For this review, take the finished solid that the model builds, in its own axes (mm). A direction names the side the tool comes from. Round coordinates to 2 decimals unless told otherwise and drop trailing zeros. Write each loop counter-clockwise with the first axis right and the second up, starting at its lowest first coordinate (ties: lowest second). Pieces come first, ordered by that corner, then holes. Notation, with made-up numbers: M 75,13.5 L 120,13.5 A18 ccw 120,20.5 Z; hole C 85,22.5 d2. An arc over 180 degrees is marked long. Use one line per item in the form item = value. Start each with the question number.
Item 1: Add section B-B (x = -9.5). State the section outline as (y, z) points.
Item 2: For P1, Ø0.8, axis at x = -20.5, z = 14.5, coming from the +Y side; P2, Ø1.5, axis at y = 2.5, z = -13.5, coming from the -X side; P3, Ø10, axis at x = -28, z = 1.5, coming from the +Y side, all flat-tipped, find the tip position at first contact; note any pin that passes through.
Item 3: For line 1 (X direction, y = 3.05, z = -2); line 2 (Z direction, x = -24.5, y = 2.1); line 3 (X direction, y = 1, z = 6), list the stretches that pass through material, from the lowest coordinate up. Write a range as [from, to].
Item 4: For faces 1 (the conical face through (-46.59, 0.54, -13.7)), 2 (the cylindrical face through (-45.4, 2.24, 15.12)), 3 (the flat face through (-20, 3, -15)), list the 3-axis set-ups (+Z, -Z, +X, -X, +Y, -Y) from which the entire face can be reached by the end or side of a thin tool; tool diameter is ignored.
Item 5: Add section A-A (z = 1). State the section outline as (x, y) points.
Item 6: Draft analysis for pull direction X (two halves, no side actions). For faces 4 (the flat face through (-49.01, 0.96, -0.14)), 5 (the flat face through (-2, 2, -0.15)), 6 (the flat face through (-21, 3, -17)), state which applies: released by +X, released by -X, zero draft, split by the parting line, or undercut.
from build123d import *

# Parameters (mm, degrees)
BOSS_EXTRUDE1_DEPTH     = 42
SKETCH3_W               = 4.5
SKETCH3_H               = 0.7
BOSS_EXTRUDE2_DEPTH     = 1.899999
SKETCH6_W               = 2.500000024
SKETCH6_H               = 0.3
REVOLVE1_ANGLE          = 90
SKETCH7_W               = 2.7
SKETCH7_H               = 5
BOSS_EXTRUDE3_DEPTH     = 2.50000008
SKETCH9_W               = 3.499999976
SKETCH9_H               = 5
CUT_EXTRUDE1_DEPTH      = 1.50000008
SKETCH10_W              = 0.3
SKETCH10_H              = 5
REVOLVE2_ANGLE          = 90
BOSS_EXTRUDE5_START     = -5
BOSS_EXTRUDE5_DEPTH     = 5
REVOLVE4_ANGLE          = 90
REVOLVE6_ANGLE          = 90
BOSS_EXTRUDE7_DEPTH     = 18
BOSS_EXTRUDE8_DEPTH     = 2.9
CUT_EXTRUDE2_DEPTH      = 2.9
BOSS_EXTRUDE9_START     = -1.899999
BOSS_EXTRUDE9_DEPTH     = 1.899999
SKETCH29_W              = 3
SKETCH29_H              = 0.9
BOSS_EXTRUDE10_DEPTH    = 1.3
CUT_EXTRUDE3_START      = -3.1
CUT_EXTRUDE3_DEPTH      = 3.1
CUT_EXTRUDE4_START      = -44.9
CUT_EXTRUDE4_DEPTH      = 2.9
SKETCH34_W              = 0.799999976
SKETCH34_H              = 5
BOSS_EXTRUDE11_DEPTH    = 2.5
CUT_EXTRUDE5_DEPTH      = 53.947521022
CUT_EXTRUDE5_DEPTH_BACK = 12.7


with BuildPart() as part:
    # Sketch1 → Boss-Extrude1 (new body)
    with BuildSketch(Plane(origin=(0, 0, 0), x_dir=(0, 0, -1), z_dir=(1, 0, 0))):
        Polygon((-4.017828461, 1.2999976), (4.017828461, 1.2999976), (7.217828411, 0.69999753), (8.7, 0.69999753), (11.9, 1.2999976), (15, 1.2999976), (15, 1.9999962), (16, 1.9999962), (16, 3.1999962), (17, 3.1999962), (17, 1.8999962), (15, 0), (-15, 0), (-17, 1.8999962), (-17, 3.1999962), (-16, 3.1999962), (-16, 1.9999962), (-15, 1.9999962), (-15, 1.2999976), (-11.9, 1.2999976), (-8.7, 0.69999753), (-7.217828411, 0.69999753), align=None)
    extrude(amount=-BOSS_EXTRUDE1_DEPTH)

    # Sketch3 → Boss-Extrude2 (add)
    with BuildSketch(Plane(origin=(0, 1.2999976, 0), x_dir=(1, 0, 0), z_dir=(0, 1, 0))):
        with Locations((-19.75, 14.65)):
            Rectangle(SKETCH3_W, SKETCH3_H)
        with Locations((-19.75, -14.65)):
            Rectangle(SKETCH3_W, SKETCH3_H)
    extrude(amount=BOSS_EXTRUDE2_DEPTH)

    # Sketch6 → Revolve1 (revolve)
    with BuildSketch(Plane(origin=(0, 1.2999976, 0), x_dir=(1, 0, 0), z_dir=(0, 1, 0))):
        with Locations((-2.249999988, 2.35)):
            Rectangle(SKETCH6_W, SKETCH6_H)
        with Locations((-2.249999988, 0)):
            Rectangle(SKETCH6_W, SKETCH6_H)
        with Locations((-2.249999988, -2.35)):
            Rectangle(SKETCH6_W, SKETCH6_H)
    revolve(axis=Axis((-0.999999976, 1.2999976, -2.5), (0, 0, -1)), revolution_arc=REVOLVE1_ANGLE)

    # Sketch20 → Revolve4 (revolve)
    with BuildSketch(Plane.ZY.offset(42)):
        Polygon((17, 3.1999962), (17, 1.8999962), (15, 0), (9, 0), (9, 0.756247537), (11.9, 0.756247537), (11.9, 1.2999976), (15, 1.2999976), (16, 1.2999976), (16, 1.9999962), (16, 3.1999962), align=None)
    revolve(axis=Axis((-42, 0, 9), (0, -1, 0)), revolution_arc=REVOLVE4_ANGLE)

    # Sketch22 → Revolve6 (revolve)
    with BuildSketch(Plane.ZY.offset(42)):
        Polygon((-9, 0.756247537), (-9, 0), (-15, 0), (-17, 1.8999962), (-17, 3.1999962), (-16, 3.1999962), (-16, 1.9999962), (-16, 1.2999976), (-15, 1.2999976), (-11.9, 1.2999976), (-11.9, 0.756247537), align=None)
    revolve(axis=Axis((-42, 3.1999962, -9), (0, 1, 0)), revolution_arc=REVOLVE6_ANGLE)

    # Sketch25 → Boss-Extrude7 (add)
    with BuildSketch(Plane.XY.offset(-9)):
        Polygon((-42, 0), (-42, 0.756247537), (-44.9, 0.756247537), (-44.9, 1.2999976), (-49, 1.2999976), (-49, 3.1999962), (-50, 3.1999962), (-50, 1.8999962), (-48, 0), align=None)
    extrude(amount=BOSS_EXTRUDE7_DEPTH)

    # Sketch26 → Boss-Extrude8 (add)
    with BuildSketch(Plane.ZY.offset(42)):
        Polygon((11.9, 0.756247537), (11.9, 1.2999976), (9, 0.756247537), align=None)
        Polygon((6.917828416, 0.756247537), (4.017828461, 1.2999976), (-4.017828461, 1.2999976), (-7.067828413, 0.728122533), align=None)
        Polygon((-9, 0.756247537), (-11.9, 1.2999976), (-11.9, 0.756247537), align=None)
    extrude(amount=BOSS_EXTRUDE8_DEPTH)

    # Sketch27 → Cut-Extrude2 (cut)
    with BuildSketch(Plane(origin=(-42, 0, 0), x_dir=(0, 0, -1), z_dir=(1, 0, 0))):
        Polygon((-8.7, 0.69999753), (-7.217828411, 0.69999753), (-6.917828416, 0.756247537), (-9, 0.756247537), align=None)
        Polygon((8.7, 0.69999753), (9, 0.756247537), (6.917828416, 0.756247537), (7.217828416, 0.69999753), align=None)
    extrude(amount=-CUT_EXTRUDE2_DEPTH, mode=Mode.SUBTRACT)

    # Sketch28 → Boss-Extrude9 (add)
    with BuildSketch(Plane(origin=(0, 3.1999962, 0), x_dir=(1, 0, 0), z_dir=(0, 1, 0)).offset(BOSS_EXTRUDE9_START)):
        Polygon((-48, 12.605551275), (-48, -12.605551275), (-48.526031835, -12.605551275), (-49.587841203, -9.896604303), (-49.587841203, 5.333499325), (-49.587841203, 9.659559889), (-49.052063671, 11.553487605), align=None)
    extrude(amount=BOSS_EXTRUDE9_DEPTH)

    # Sketch29 → Boss-Extrude10 (add)
    with BuildSketch(Plane(origin=(-48, 0, 0), x_dir=(0, 0, -1), z_dir=(1, 0, 0))):
        with Locations((6.5, 2.7499962)):
            Rectangle(SKETCH29_W, SKETCH29_H)
        with Locations((-6.5, 2.7499962)):
            Rectangle(SKETCH29_W, SKETCH29_H)
    extrude(amount=BOSS_EXTRUDE10_DEPTH)

    # Sketch31 → Cut-Extrude3 (cut)
    with BuildSketch(Plane(origin=(-44.9, 0, 0), x_dir=(0, 0, -1), z_dir=(1, 0, 0)).offset(CUT_EXTRUDE3_START)):
        Polygon((-8.7, 0.69999753), (-7.217828411, 0.69999753), (-4.017828461, 1.2999976), (-9, 1.2999976), (-11.9, 1.2999976), align=None)
        Polygon((4.017828461, 1.2999976), (7.217828416, 0.69999753), (8.7, 0.69999753), (11.9, 1.2999976), align=None)
    extrude(amount=CUT_EXTRUDE3_DEPTH, mode=Mode.SUBTRACT)

    # Sketch33 → Cut-Extrude4 (cut)
    with BuildSketch(Plane(origin=(0, 0, 0), x_dir=(0, 0, -1), z_dir=(1, 0, 0)).offset(CUT_EXTRUDE4_START)):
        Polygon((-11.9, 1.2999976), (-4.017828461, 1.2999976), (-7.217828411, 0.69999753), (-8.7, 0.69999753), align=None)
        Polygon((4.017828461, 1.2999976), (11.9, 1.2999976), (8.7, 0.69999753), (7.272372627, 0.69999753), align=None)
    extrude(amount=CUT_EXTRUDE4_DEPTH, mode=Mode.SUBTRACT)



with BuildPart() as body_2:
    # Sketch7 → Boss-Extrude3 (new body)
    with BuildSketch(Plane(origin=(1.692653476, 1.2999976, 1.325896357), x_dir=(1, 0, 0), z_dir=(0, 1, 0))):
        with Locations((-0.542653476, 1.325896357)):
            Rectangle(SKETCH7_W, SKETCH7_H)
    extrude(amount=BOSS_EXTRUDE3_DEPTH)

    # Sketch9 → Cut-Extrude1 (cut)
    with BuildSketch(Plane.XZ.offset(-1.2999976)):
        with Locations((0.750000012, 0)):
            Rectangle(SKETCH9_W, SKETCH9_H)
    extrude(amount=-CUT_EXTRUDE1_DEPTH, mode=Mode.SUBTRACT)

    # Sketch10 → Revolve2 (revolve)
    with BuildSketch(Plane.XZ.offset(-2.79999768)):
        with Locations((1.15, 0)):
            Rectangle(SKETCH10_W, SKETCH10_H)
    revolve(axis=Axis((1.3, 2.79999768, 2.5), (0, 0, 1)), revolution_arc=REVOLVE2_ANGLE)

    # Sketch11 → Boss-Extrude5 (add)
    with BuildSketch(Plane(origin=(0, 0, -2.5), x_dir=(-1, 0, 0), z_dir=(0, 0, -1)).offset(BOSS_EXTRUDE5_START)):
        Polygon((-1.3, 2.49999768), (-2.5, 2.79999768), (-1.3, 2.79999768), align=None)
    extrude(amount=BOSS_EXTRUDE5_DEPTH)


with BuildPart() as part_1:
    add(part.part)

    add(body_2.part)  # Boss-Extrude11 merges body 2
    # Sketch34 → Boss-Extrude11 (add)
    with BuildSketch(Plane(origin=(0, 1.2999976, 0), x_dir=(1, 0, 0), z_dir=(0, 1, 0))):
        with Locations((-0.599999988, 0)):
            Rectangle(SKETCH34_W, SKETCH34_H)
    extrude(amount=BOSS_EXTRUDE11_DEPTH)

    # Sketch36 → Cut-Extrude5 (cut, two sides: drawn at the far end of the back side and taken through both)
    with BuildSketch(Plane.XY.offset(-CUT_EXTRUDE5_DEPTH_BACK)):
        Polygon((-50, 1.8999962), (-48, 0), (-50, 0), align=None)
    extrude(amount=CUT_EXTRUDE5_DEPTH + CUT_EXTRUDE5_DEPTH_BACK, mode=Mode.SUBTRACT)


solid = part_1.part
Calculated:
q1.outline = M 0,-15 L 1.9,-17 L 3.2,-17 L 3.2,-16 L 2,-16 L 2,-15 L 1.3,-15 L 1.3,-11.9 L 0.7,-8.7 L 0.7,-7.22 L 1.3,-4.02 L 1.3,4.02 L 0.7,7.22 L 0.7,8.7 L 1.3,11.9 L 1.3,15 L 2,15 L 2,16 L 3.2,16 L 3.2,17 L 1.9,17 L 0,15 Z
q2.P1 = 3.2
q2.P2 = -49.07
q2.P3 = 1.3
q3.line_1 = [-50, -48], [-1, 2.5]
q3.line_2 = [-17, -16], [16, 17]
q3.line_3 = [-49.05, -48]
q4.face_1 = -Z, -X, -Y
q4.face_2 = +Y
q4.face_3 = +X, +Y
q5.outline = M -50,1.9 L -48,0 L 0,0 L 0,1.3 L -0.2,1.3 L -0.2,2.8 L 1,2.8 A0.3 ccw 1.3,2.5 L 2.5,2.8 L 2.5,3.8 L -1,3.8 L -1,1.3 L -48,1.3 L -48,3.2 L -50,3.2 Z
q6.face_4 = released by -X
q6.face_5 = undercut
q6.face_6 = zero draft
